CAD build for the part. Positions are in the model's coordinates, mm. Face numbers are marked on the shaded views. A direction names the side the tool comes from. Give positions to 0.01 mm unless a question says otherwise; leave off trailing zeros. Loops run counter-clockwise (first coordinate to the right, second up) from the corner with the lowest first, then second, coordinate; pieces in that order, holes last. Notation, with made-up numbers: M -19,25.5 L 8,25.5 A14 cw 8,51.5 Z; hole C 46.25,14.25 d9. An arc over 180 degrees is marked long. Answer as CSV lines item,"result".
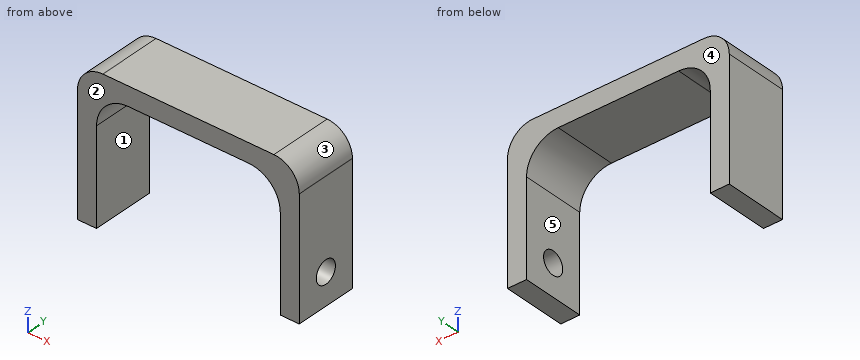
```python
from build123d import *

# Parameters (mm, degrees)
CYLINDER001_R     = 1.8
CYLINDER001_DEPTH = 40
PAD001_DEPTH      = 10


with BuildPart() as hole001:
    # Cylinder001 → Cylinder001 (new body)
    with BuildSketch(Plane(origin=(-4, -5, 5), x_dir=(0, 0, -1), z_dir=(1, 0, 0))):
        Circle(CYLINDER001_R)
    extrude(amount=CYLINDER001_DEPTH)


with BuildPart() as cut001:
    # Sketch001 → Pad001 (new body)
    with BuildSketch(Plane.XZ):
        with BuildLine():
            Line((-14.5, 0), (-14.5, 15))
            ThreePointArc((-9.5, 20), (-13.035534, 18.535534), (-14.5, 15))
            Line((-9.5, 20), (9.5, 20))
            ThreePointArc((14.5, 15), (13.035534, 18.535534), (9.5, 20))
            Line((14.5, 15), (14.5, 0))
            Line((17.5, 0), (14.5, 0))
            Line((17.5, 19), (17.5, 0))
            ThreePointArc((17.5, 19), (16.328427, 21.828427), (13.5, 23))
            Line((-13.5, 23), (13.5, 23))
            ThreePointArc((-13.5, 23), (-16.328427, 21.828427), (-17.5, 19))
            Line((-17.5, 0), (-17.5, 19))
            Line((-14.5, 0), (-17.5, 0))
        make_face()
    extrude(amount=PAD001_DEPTH)

    # Cut001: cut hole001
    add(hole001.part, mode=Mode.SUBTRACT)


solid = cut001.part
```
Q1. Cut at A-A (y = -5). Write the cut outline in (x, z).
Solution:
outline,"M -17.5,0 L -14.5,0 L -14.5,15 A5 cw -9.5,20 L 9.5,20 A5 cw 14.5,15 L 14.5,6.8 L 17.5,6.8 L 17.5,19 A4 ccw 13.5,23 L -13.5,23 A4 ccw -17.5,19 Z; M 14.5,0 L 17.5,0 L 17.5,3.2 L 14.5,3.2 Z"
Q2. Wall check: line 1 (X direction, y = -7.75, z = 8.75); line 2 (Y direction, x = 15.7, z = 5); line 3 (Z direction, x = 1.5, y = -5). Give the ranges that are in metal, low to high. Write a range as [from, to].
Solution:
line 1,"x = [-17.5, -14.5], [14.5, 17.5]"
line 2,"y = [-10, -6.8], [-3.2, 0]"
line 3,"z = [20, 23]"
Q3. Which spindle directions (+Z, -Z, +X, -X, +Y, -Y) get a long thin tool onto all of the face, cutting with end or side? Do the marked faces 1 and 2. Say none if no direction does.
Solution:
face 1,"-Z, +Y, -Y"
face 2,"+Z, -Z, +X, -X, -Y"
Q4. Cut at B-B (z = 18). Write the cut outline in (x, y), and give its area (3 significant figures).
Solution:
outline,"M -17.5,-10 L -13.5,-10 L -13.5,0 L -17.5,0 Z; M 13.5,-10 L 17.5,-10 L 17.5,0 L 13.5,0 Z"
area,"80.0 mm²"
Q5. Cut at C-C (z = 5). Write the cut outline in (x, y), and give its area (3 significant figures).
Solution:
outline,"M -17.5,-10 L -14.5,-10 L -14.5,0 L -17.5,0 Z; M 14.5,-10 L 17.5,-10 L 17.5,-6.8 L 14.5,-6.8 Z; M 14.5,-3.2 L 17.5,-3.2 L 17.5,0 L 14.5,0 Z"
area,"49.2 mm²"
Q6. Mould opens along X. For the marked faces 3, 4 and 5 say: released by +X, released by -X, zero draft, split by the parting line, or undercut.
Solution:
face 3,"released by +X"
face 4,"zero draft"
face 5,"undercut"
Q7. Cut at D-D (y = -1.5). Write the cut outline in (x, z).
Solution:
outline,"M -17.5,0 L -14.5,0 L -14.5,15 A5 cw -9.5,20 L 9.5,20 A5 cw 14.5,15 L 14.5,0 L 17.5,0 L 17.5,19 A4 ccw 13.5,23 L -13.5,23 A4 ccw -17.5,19 Z"
